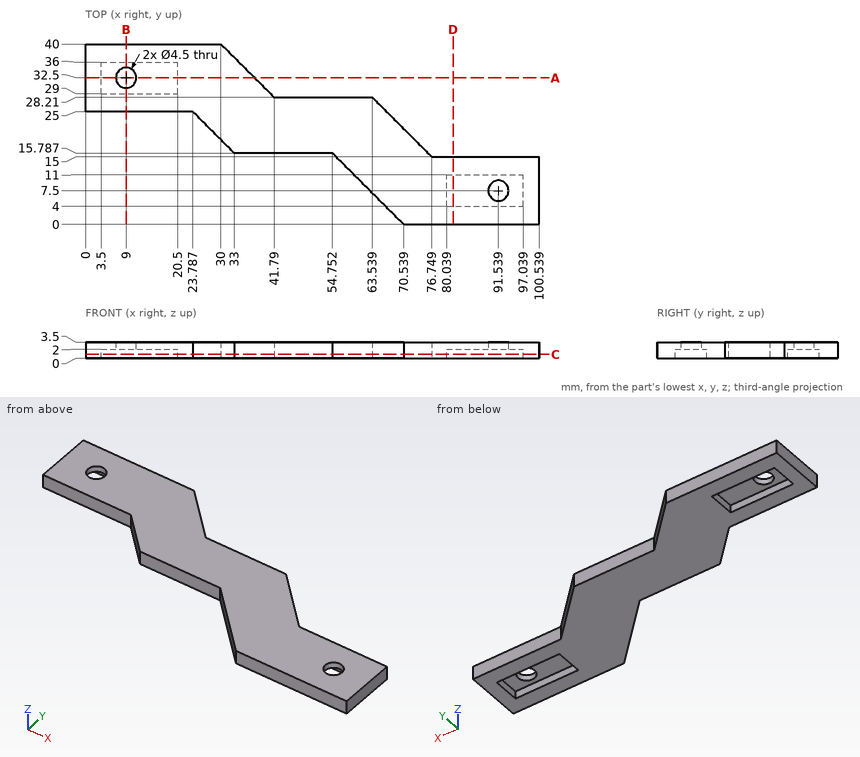
Design review of the part shown in the three views and the two pictorial views. Dimensions are in mm from the part's minimum x, y and z. Round coordinates to 2 decimals unless told otherwise and drop trailing zeros. Order: outer loops, then holes, each group sorted by start corner. A loop starts at its lowest first (then second) coordinate and runs counter-clockwise, first axis right, second up. Notation, with made-up numbers: M 58,63.5 L 114,63.5 A31 cw 114,88.5 Z; hole C -3.75,-24 d10. An arc over 180 degrees is marked long. Put each result on its own line as item: value.
Q1. Consider section C-C (z = 0.85). State the section outline as (x, y) points, and give its area (3 significant figures).
Reported:
outline: M 0,25 L 23.79,25 L 33,15.79 L 54.75,15.79 L 70.54,0 L 100.54,0 L 100.54,15 L 76.75,15 L 63.54,28.21 L 41.79,28.21 L 30,40 L 0,40 Z; hole M 3.5,29 L 20.5,29 L 20.5,36 L 3.5,36 Z; hole M 80.04,4 L 97.04,4 L 97.04,11 L 80.04,11 Z
area: 1,370 mm²
Q2. Consider section B-B (x = 9). State the section outline as (y, z) points.
Reported:
outline: M 25,0 L 29,0 L 29,2 L 30.25,2 L 30.25,3.5 L 25,3.5 Z; M 34.75,2 L 36,2 L 36,0 L 40,0 L 40,3.5 L 34.75,3.5 Z
Q3. Consider section A-A (y = 32.5). State the section outline as (x, z) points.
Reported:
outline: M 0,0 L 3.5,0 L 3.5,2 L 6.75,2 L 6.75,3.5 L 0,3.5 Z; M 11.25,2 L 20.5,2 L 20.5,0 L 37.5,0 L 37.5,3.5 L 11.25,3.5 Z
Q4. To check wall thickness, follow line 1 (Y direction, x = 7, z = 1.9); line 2 (Y direction, x = 79.5, z = 1.2); line 3 (Y direction, x = 42, z = 0.5). State the ranges of each line that lie inside material, in increasing order.
Reported:
line 1: 25 to 29, 36 to 40
line 2: 0 to 15
line 3: 15.79 to 28.21
Q5. Insertion check: pin 1 Ø1.6 at (y, z) = (8.5, 1.5) entering from -X; pin 2 Ø1.8 at (x, z) = (88, 2) entering from +Y; pin 3 Ø0.6 at (x, z) = (8, 1) entering from -Y; pin 4 Ø5.5 at (x, y) = (8.5, 31) entering from -Z. Each pin has a flat end and moves straight along its axis. Give the tip position at first contact, or say it passes through.
Reported:
pin 1: x = 61.24
pin 2: y = 15
pin 3: y = 25
pin 4: z = 0
Q6. Consider section D-D (x = 81.5). State the section outline as (y, z) points, and give its area (3 significant figures).
Reported:
outline: M 0,0 L 4,0 L 4,2 L 11,2 L 11,0 L 15,0 L 15,3.5 L 0,3.5 Z
area: 38.5 mm²
